Source: three-view drawing plus pictorial views. Frame: mm from the lowest corner of the part. A direction names the side the tool comes from. Coordinates: 2 decimals unless noted, no trailing zeros. Write each loop counter-clockwise with the first axis right and the second up, starting at its lowest first coordinate (ties: lowest second). Pieces come first, ordered by that corner, then holes. Notation, with made-up numbers: (20.25, 45.5) - (69.25, 45.5) arc R17 cw to (69.25, 49.5) - close; hole circle Ø11 at (-33.5, 73.25). An arc over 180 degrees is marked (long way). Put each result on its own line as item: value.
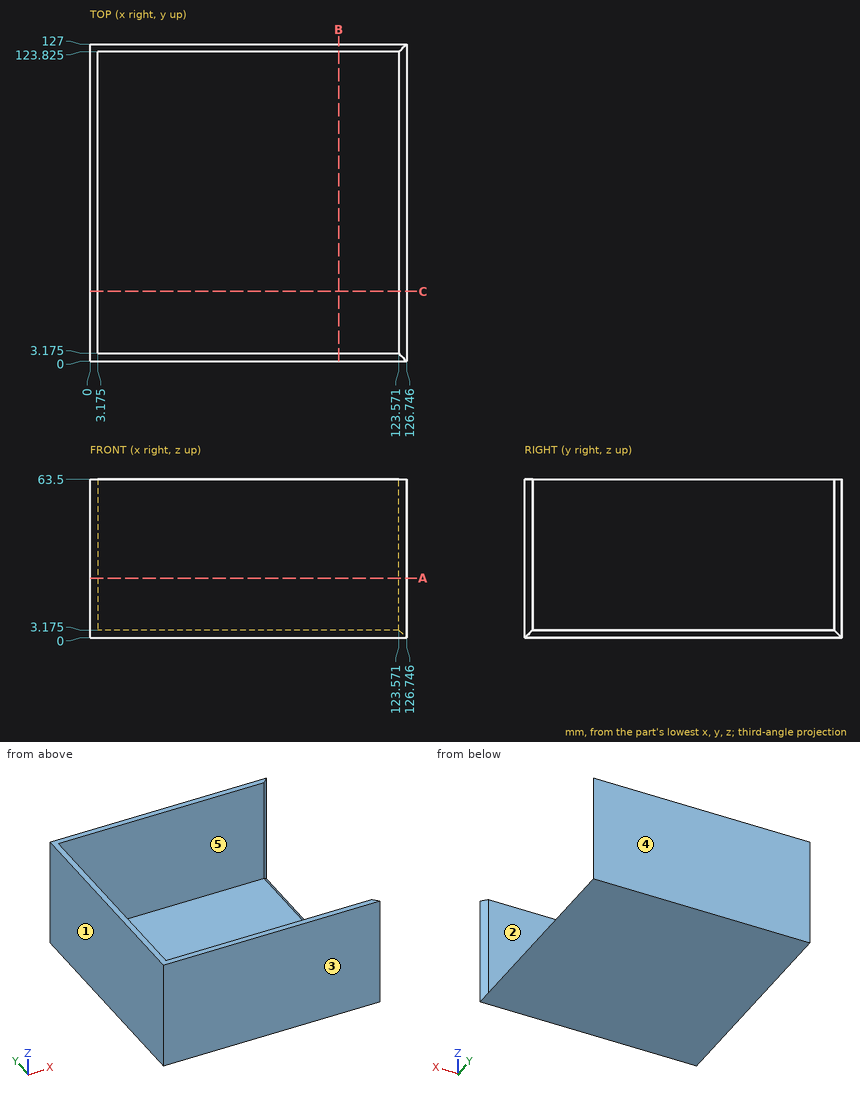
1. Pin query (flat end, axial travel): pin 1 Ø3 at (y, z) = (87, 27) entering from +X (3 decimals). Return the tip coordinate at first contact, or that it passes through.
Answer below:
pin 1: stops at x = 3.175
2. Mould query, pull axis Y, two halves, no side actions, for the marked faces 1, 2 and 3. Classes: +Y half, -Y half, draft (parallel to the pull), parting line (faces both ways), or undercut.
Answer below:
face 1: draft
face 2: undercut
face 3: -Y half
3. Set-up query: the marked faces 4 and 5. Return all of +Z, -Z, +X, -X, +Y, -Y with unobstructed straight access to the full face (end or side cutting, diameter ignored); none if empty.
Answer below:
face 4: +Z, -Z, +X, -X, +Y
face 5: +Z, +X
4. Section query C-C (y = 28). Return loops of the section in (x, z) (3 decimals).
Answer below:
outline: (0, 0) - (126.746, 0) - (123.571, 3.175) - (3.175, 3.175) - (3.175, 63.5) - (0, 63.5) - close
5. Section query B-B (x = 99.5). Return loops of the section in (y, z) (3 decimals), then the cut area to 3 significant figures.
Answer below:
outline: (0, 0) - (127, 0) - (127, 63.5) - (123.825, 63.5) - (123.825, 3.175) - (3.175, 3.175) - (3.175, 63.5) - (0, 63.5) - close
area: 786 mm²
6. Ray query, probe 1 along Y at (x, z) = (9, 59) (3 decimals); probe 2 along Z at (x, y) = (81.5, 32.5) (3 decimals). Return the intervals inside material, ascending. Write a range as from..to.
Answer below:
probe 1: y = 0..3.175, 123.825..127
probe 2: z = 0..3.175
7. Section query A-A (z = 24). Return loops of the section in (x, y) (3 decimals), then the cut area to 3 significant figures.
Answer below:
outline: (0, 0) - (126.746, 0) - (123.571, 3.175) - (3.175, 3.175) - (3.175, 123.825) - (123.571, 123.825) - (126.746, 127) - (0, 127) - close
area: 1,180 mm²
